```python
from build123d import *

# Parameters (mm, degrees)
F0_W         = 12.7
F0_H         = 12.7
F1_DEPTH     = 25.4
F2_R         = 5.5626
F3_DEPTH     = 19.05
F4_W         = 3.0250146519
F4_H         = 2.872077981
F5_DEPTH     = 12.7
F7_DEPTH     = 2.8448
F8_R         = 1.016
F9_DEPTH     = 5.2832
F10_T1_DEPTH = 4.6143001951
F10_T3_DEPTH = 4.6143001951


# Not quite as in the source:
# - a fillet or chamfer that OpenCascade refuses, or shapes differently, is made with other operations: its cross-section is extruded or revolved along the edge and cut away or added


with BuildPart() as f1:
    # F0 (on Right) → F1 (new body)
    with BuildSketch(Plane.YZ):
        Rectangle(F0_W, F0_H)
    extrude(amount=-F1_DEPTH)

    # F2 (on face) → F3 (cut)
    with BuildSketch(Plane(origin=(-25.4, 0, 0), x_dir=(0, -1, 0), z_dir=(-1, 0, 0))):
        Circle(F2_R)
    extrude(amount=-F3_DEPTH, mode=Mode.SUBTRACT)

    # F4 (on face) → F5 (join)
    with BuildSketch(Plane.YZ):
        Rectangle(F4_W, F4_H)
    extrude(amount=F5_DEPTH)

    # F6 (on face) → F7 (join)
    with BuildSketch(Plane(origin=(0, 0, -1.4360389905), x_dir=(1, 0, 0), z_dir=(0, 0, -1))):
        Polygon((12.0346518233, 3.5868075211), (12.0346518233, 1.512507326), (12.7, 1.512507326), (18.0126260966, 1.512507326), (18.0126260966, 3.5868075211), align=None)
        Polygon((18.0126260966, -1.512507326), (12.7, -1.512507326), (12.0346518233, -1.512507326), (12.0346518233, -3.5868075211), (18.0126260966, -3.5868075211), align=None)
    extrude(amount=-F7_DEPTH)

    # F8 (on face) → F9 (join)
    with BuildSketch(Plane.XZ.offset(3.5868075211)):
        with Locations((15.02363896, 0)):
            Circle(F8_R)
    extrude(amount=-F9_DEPTH)

    # F10: fillet of radius 0.508 on 4 edges, made by hand

    # F10_s2 → F10_t1 (cut)
    with BuildSketch(Plane.XZ.offset(0.242507326)):
        with BuildLine():
            add(Edge.make_bspline(
                [(17.5046260966, -1.4360389905), (18.0126260966, -1.4360389905), (18.0126260966, -0.9280389905)],
                knots=[0, 0, 0, 1, 1, 1], degree=2, weights=[1, 1, 1]))
            Line((18.0126260966, -0.9280389905), (18.0126260966, -1.4360389905))
            Line((18.0126260966, -1.4360389905), (17.5046260966, -1.4360389905))
        make_face()
        with BuildLine():
            add(Edge.make_bspline(
                [(18.0126260966, 0.9007610095), (18.0126260966, 1.4087610095), (17.5046260966, 1.4087610095)],
                knots=[0, 0, 0, 1, 1, 1], degree=2, weights=[1, 1, 1]))
            Line((17.5046260966, 1.4087610095), (18.0126260966, 1.4087610095))
            Line((18.0126260966, 1.4087610095), (18.0126260966, 0.9007610095))
        make_face()
    extrude(amount=F10_T1_DEPTH, mode=Mode.SUBTRACT)

    # F10_s4 → F10_t3 (cut)
    with BuildSketch(Plane.XZ.offset(-4.8568075211)):
        with BuildLine():
            add(Edge.make_bspline(
                [(17.5046260966, -1.4360389905), (18.0126260966, -1.4360389905), (18.0126260966, -0.9280389905)],
                knots=[0, 0, 0, 1, 1, 1], degree=2, weights=[1, 1, 1]))
            Line((18.0126260966, -0.9280389905), (18.0126260966, -1.4360389905))
            Line((18.0126260966, -1.4360389905), (17.5046260966, -1.4360389905))
        make_face()
        with BuildLine():
            add(Edge.make_bspline(
                [(18.0126260966, 0.9007610095), (18.0126260966, 1.4087610095), (17.5046260966, 1.4087610095)],
                knots=[0, 0, 0, 1, 1, 1], degree=2, weights=[1, 1, 1]))
            Line((17.5046260966, 1.4087610095), (18.0126260966, 1.4087610095))
            Line((18.0126260966, 1.4087610095), (18.0126260966, 0.9007610095))
        make_face()
    extrude(amount=F10_T3_DEPTH, mode=Mode.SUBTRACT)


solid = f1.part
```
Check sheet for the modelled part. Datum: model origin and axes. Units: mm. A direction names the side the tool comes from. Give positions to 0.01 mm unless a question says otherwise; leave off trailing zeros. Write each loop counter-clockwise with the first axis right and the second up, starting at its lowest first coordinate (ties: lowest second). Pieces come first, ordered by that corner, then holes. Notation, with made-up numbers: (76, -33) - (107, -33) arc R33 cw to (107, 0) - close; hole circle Ø11 at (12, 44). An arc over 180 degrees is marked (long way). Answer as a JSON object with one key per item and string values. Group by question number.
1) Sectioned sample at A-A (y = 0). Record the cut outline in (x, z), then the cut area to 3 significant figures.
2) Depth check by flat-ended pin: P1, Ø3, axis at x = 16.5, z = 0, coming from the -Y side; P2, Ø1, axis at y = 2, z = 0, coming from the -X side; P3, Ø3, axis at x = 6.5, z = -0.5, coming from the +Y side. Enter the tip coordinate at first touch or a pass-through.
3) Release check for a two-part mould opening along Y. For faces 1 (the face through (-13, 6.35, 0)), 2 (the face through (-13, -6.35, 0)), 3 (the face through (18.013, -3, 0)), 4 (the face through (-16.008, -5.306, 1.671)) record: pulls with the +Y half, pulls with the -Y half, needs draft (parallel to the pull), parting line crosses it, or undercut.
4) Sectioned sample at C-C (x = -13.5). Record the cut outline in (y, z), then the cut area to 3 significant figures.
5) Sectioned sample at D-D (z = 3.5). Record the cut outline in (x, y), then the cut area to 3 significant figures.
6) Sectioned sample at B-B (z = 0). Record the cut outline in (x, y).
7) Thickness scan on probe 1 along Z at (x, y) = (-21, 0); probe 2 along X at (y, z) = (3.5, -0.5); probe 3 along X at (y, z) = (-0.5, 3.25). Record the ranges inside material, lowest first. Write a range as from..to.
8) Access from +Z, -Z, +X, -X, +Y, -Y to the whole of each face (thin tool, end or side, straight path). Record for faces 5 (the face through (12.035, 3, 0)), 6 (the face through (12.035, -3, 0)), 7 (the face through (-6.35, 0, 0)), 8 (the face through (15, -3.587, 0)).
Geometry results:
{
 "1": {"outline": "(-25.4, -6.35) - (0, -6.35) - (0, -1.44) - (12.7, -1.44) - (12.7, 1.44) - (0, 1.44) - (0, 6.35) - (-25.4, 6.35) - (-25.4, 5.56) - (-6.35, 5.56) - (-6.35, -5.56) - (-25.4, -5.56) - close; circle Ø2.03 at (15.02, 0)", "area": "150 mm^2"},
 "2": {"P1": "stops at y = -3.59", "P2": "stops at x = -6.35", "P3": "stops at y = 1.51"},
 "3": {"face 1": "pulls with the +Y half", "face 2": "pulls with the -Y half", "face 3": "needs draft", "face 4": "undercut"},
 "4": {"outline": "(-6.35, -6.35) - (6.35, -6.35) - (6.35, 6.35) - (-6.35, 6.35) - close; hole circle Ø11.13 at (0, 0)", "area": "64.1 mm^2"},
 "5": {"outline": "(-25.4, -6.35) - (0, -6.35) - (0, 6.35) - (-25.4, 6.35) - (-25.4, 4.32) - (-6.35, 4.32) - (-6.35, -4.32) - (-25.4, -4.32) - close", "area": "158 mm^2"},
 "6": {"outline": "(-25.4, -6.35) - (0, -6.35) - (0, -1.51) - (12.03, -1.51) - (12.03, -3.59) - (18.01, -3.59) - (18.01, -1.51) - (16.04, -1.51) - (16.04, 1.51) - (18.01, 1.51) - (18.01, 3.59) - (12.03, 3.59) - (12.03, 1.51) - (0, 1.51) - (0, 6.35) - (-25.4, 6.35) - (-25.4, 5.56) - (-6.35, 5.56) - (-6.35, -5.56) - (-25.4, -5.56) - close; hole (12.7, -1.51) - (14.01, -1.51) - (14.01, 1.51) - (12.7, 1.51) - close"},
 "7": {"probe 1": "z = -6.35..-5.56, 5.56..6.35", "probe 2": "x = -6.35..0, 12.03..18.01", "probe 3": "x = -6.35..0"},
 "8": {"face 5": "+Z, -Z, +Y", "face 6": "+Z, -Z, -Y", "face 7": "-X", "face 8": "+Z, -Z, +X, -Y"}
}
